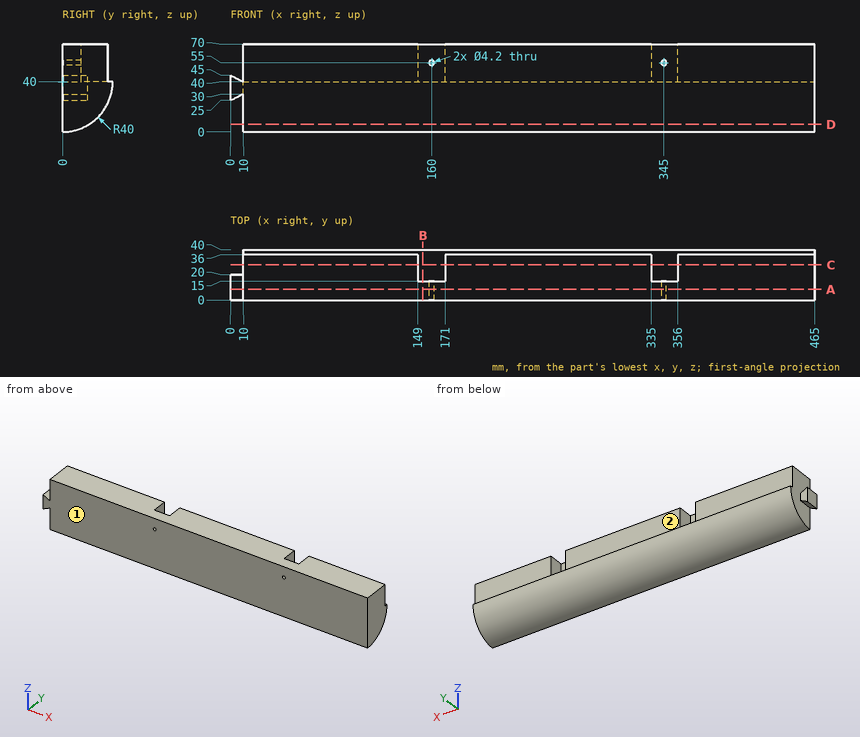
Job drawing, mm, ordinate dimensions from the low corner. One solid piece. A direction names the side the tool comes from. Give positions to 0.01 mm unless a question says otherwise; leave off trailing zeros. Write each loop counter-clockwise with the first axis right and the second up, starting at its lowest first coordinate (ties: lowest second). Pieces come first, ordered by that corner, then holes. Notation, with made-up numbers: (69, -3.5) -> (106, -3.5) arc R21 ccw to (106, 5.5) -> close; hole circle Ø5 at (85, 29). An arc over 180 degrees is marked (long way). Return JSON: item names as keys, results as strings.
Item 1: Band-saw the part on C-C (y = 28). List the corners of the cut face in (x, z), then the cut area to 3 significant figures.
Answer below:
{"outline": "(10, 11.43) -> (465, 11.43) -> (465, 70) -> (356, 70) -> (356, 40) -> (335, 40) -> (335, 70) -> (171, 70) -> (171, 40) -> (149, 40) -> (149, 70) -> (10, 70) -> close", "area": "25,400 mm2"}
Item 2: Band-saw the part on B-B (x = 153). List the corners of the cut face in (y, z), then the cut area to 3 significant figures.
Answer below:
{"outline": "(0, 0) arc R40 ccw to (40, 40) -> (15, 40) -> (15, 70) -> (0, 70) -> close", "area": "1,710 mm2"}
Item 3: Drill centre lines: probe 1 along X at (y, z) = (19.5, 57); probe 2 along X at (y, z) = (28, 28); probe 3 along Y at (x, z) = (399.5, 43). Where is each one in solid material? Low to high.
Answer below:
{"probe 1": "x = 10 to 149, 171 to 335, 356 to 465", "probe 2": "x = 10 to 465", "probe 3": "y = 0 to 36"}
Item 4: Drop flat-ended pins along their axis: pin 1 (10 mm diameter, centred on x = 81.5, z = 27, fed in from +Y); pin 2 (4 mm diameter, centred on x = 189.5, z = 53, fed in from +Y); pin 3 (5 mm diameter, centred on x = 160, z = 55, fed in from +Y). Give the stop position or say it passes through.
Answer below:
{"pin 1": "stops at y = 39.19", "pin 2": "stops at y = 36", "pin 3": "stops at y = 15"}
Item 5: Band-saw the part on D-D (z = 6). List the corners of the cut face in (x, y), then the cut area to 3 significant figures.
Answer below:
{"outline": "(10, 0) -> (465, 0) -> (465, 21.07) -> (10, 21.07) -> close", "area": "9,590 mm2"}
Item 6: Tool access for the marked faces 1 and 2: list every direction of +Z, -Z, +X, -X, +Y, -Y with a clear straight run to the whole face (end or side of a thin tool).
Answer below:
{"face 1": "+Z, -Z, +X, -X, -Y", "face 2": "+Z, +X, -X, +Y"}
Item 7: Band-saw the part on A-A (y = 8.5). List the corners of the cut face in (x, z).
Answer below:
{"outline": "(0, 25) -> (10, 30) -> (10, 0.91) -> (465, 0.91) -> (465, 70) -> (10, 70) -> (10, 40) -> (0, 45) -> close; hole circle Ø4.2 at (160, 55); hole circle Ø4.2 at (345, 55)"}
